Read the model definition and answer for the solid it produces. Units are mm, in the model's axes. Face numbers are marked on the shaded views. Round coordinates to 2 decimals unless told otherwise and drop trailing zeros. Order: outer loops, then holes, each group sorted by start corner. A loop starts at its lowest first (then second) coordinate and runs counter-clockwise, first axis right, second up. Notation, with made-up numbers: (22, 88.25) - (58, 88.25) arc R17 cw to (58, 110.25) - close; hole circle Ø6 at (72.25, 54.25). An arc over 180 degrees is marked (long way). Answer as a JSON object with one key per item and string values. Group by question number.
Q1. A cutting plane is placed at B-B on x = -9.5. Determine the outline of the cut face in (y, z), and give its area (3 significant figures).
Q2. The mould has two halves that part along Y. Classify the marked faces 1, 2 and 3: pulls with the +Y half, pulls with the -Y half, needs draft (parallel to the pull), parting line crosses it, or undercut.
Q3. A cutting plane is placed at D-D on z = 2.45. Determine the outline of the cut face in (x, y), and give its area (3 significant figures).
Q4. A cutting plane is placed at C-C on y = 1. Count the separate pieces of the cut face and the enclosed holes in it, and give its area (3 significant figures).
Q5. Consider line 1 (X direction, y = 0.5, z = 2.4); line 2 (Y direction, x = -15, z = 1.6); line 3 (X direction, y = 0.5, z = 1.15). Determine where each line is inside the solid, lowest interval first.
Q6. Given pin 1 Ø4 at (x, y) = (-15, 0) entering from -Z; pin 2 Ø2 at (x, y) = (0, 0) entering from +Z, each flat-ended and moving along its own axis, determine where each tip first touches the part or whether it passes through.
Q7. A cutting plane is placed at A-A on z = 1.55. Determine the outline of the cut face in (x, y), and give its area (3 significant figures).
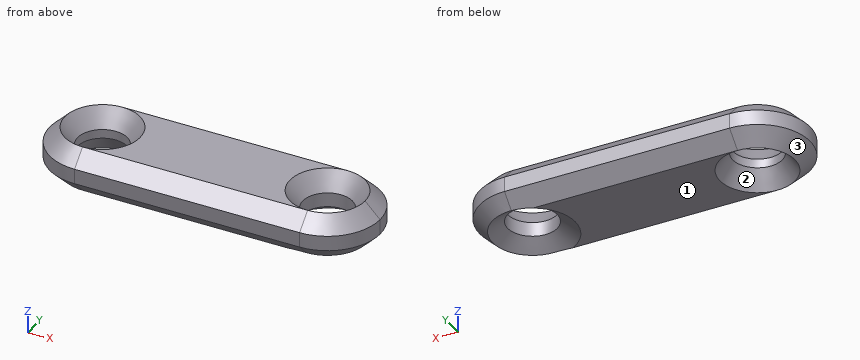
```python
from build123d import *

# Parameters (mm, degrees)
F0_R     = 1.65
F1_DEPTH = 3
F2_SIZE  = 1


# Not quite as in the source:
# - a fillet or chamfer that OpenCascade refuses, or shapes differently, is made with other operations: its cross-section is extruded or revolved along the edge and cut away or added


with BuildPart() as f1:
    # F0 (on Top) → F1 (new body)
    with BuildSketch(Plane.XY):
        with BuildLine():
            ThreePointArc((-15, -3.5), (-12.5251262658, -2.4748737342), (-11.5, 0))
            ThreePointArc((-11.5, 0), (-12.5251262658, 2.4748737342), (-15, 3.5))
            ThreePointArc((-15, 3.5), (-18.5, 0), (-15, -3.5))
        make_face()
        with Locations((-15, 0)):
            Circle(F0_R, mode=Mode.SUBTRACT)
        with BuildLine():
            ThreePointArc((-15, 3.5), (-12.5251262658, 2.4748737342), (-11.5, 0))
            ThreePointArc((-11.5, 0), (-12.5251262658, -2.4748737342), (-15, -3.5))
            Line((-15, -3.5), (0, -3.5))
            ThreePointArc((0, -3.5), (-3.5, 0), (0, 3.5))
            Line((0, 3.5), (-15, 3.5))
        make_face()
        with BuildLine():
            ThreePointArc((3.5, 0), (2.4748737342, 2.4748737342), (0, 3.5))
            ThreePointArc((0, 3.5), (-3.5, 0), (0, -3.5))
            ThreePointArc((0, -3.5), (2.4748737342, -2.4748737342), (3.5, 0))
        make_face()
        Circle(F0_R, mode=Mode.SUBTRACT)
    extrude(amount=F1_DEPTH)

    # F2
    f2_edges = [f1.edges().sort_by_distance(p)[0] for p in [
        (-7.5, -3.5, 3),
        (-18.5, 0, 3),
        (3.5, 0, 3),
        (-7.5, 3.5, 3),
        (-7.5, -3.5, 0),
        (-18.5, 0, 0),
        (3.5, 0, 0),
        (-7.5, 3.5, 0),
    ]]
    chamfer(f2_edges, length=F2_SIZE)

    # F3: chamfer of 1.2 x 0.85 on 4 edges, made by hand

    # F3_s1 → F3_t2 (revolve, cut)
    with BuildSketch(Plane.XZ):
        Polygon((-12.5, 3), (-13.35, 1.8), (-13.35, 3), align=None)
    revolve(axis=Axis((-15, 0, 3), (0, 0, 1)), mode=Mode.SUBTRACT)

    # F3_s3 → F3_t4 (revolve, cut)
    with BuildSketch(Plane.XZ):
        Polygon((2.5, 3), (1.65, 1.8), (1.65, 3), align=None)
    revolve(axis=Axis((0, 0, 3), (0, 0, 1)), mode=Mode.SUBTRACT)

    # F3_s5 → F3_t6 (revolve, cut)
    with BuildSketch(Plane.XZ):
        Polygon((2.85, 0), (1.65, 0.85), (1.65, 0), align=None)
    revolve(axis=Axis((0, 0, 0), (0, 0, 1)), mode=Mode.SUBTRACT)

    # F3_s7 → F3_t8 (revolve, cut)
    with BuildSketch(Plane.XZ):
        Polygon((-12.5, 0), (-13.35, 1.2), (-13.35, 0), align=None)
    revolve(axis=Axis((-15, 0, 0), (0, 0, 1)), mode=Mode.SUBTRACT)


solid = f1.part
```
Result set:
{
 "1": {"outline": "(-3.5, 1) - (-2.5, 0) - (2.5, 0) - (3.5, 1) - (3.5, 2) - (2.5, 3) - (-2.5, 3) - (-3.5, 2) - close", "area": "19.0 mm²"},
 "2": {"face 1": "needs draft", "face 2": "undercut", "face 3": "parting line crosses it"},
 "3": {"outline": "(-15, -3.05) - (0, -3.05) arc R3.05 ccw to (0, 3.05) - (-15, 3.05) arc R3.05 ccw to start; hole circle Ø4.22 at (-15, 0); hole circle Ø4.22 at (0, 0)", "area": "92.7 mm²"},
 "4": {"separate pieces": "3", "enclosed holes": "0", "area": "42.5 mm²"},
 "5": {"line 1": "x = -18.06 to -17.01, -12.99 to -2.01, 2.01 to 3.06", "line 2": "y = -3.5 to -1.65, 1.65 to 3.5", "line 3": "x = -18.46 to -16.61, -13.39 to -1.57, 1.57 to 3.46"},
 "6": {"pin 1": "stops at z = 0.71", "pin 2": "passes through"},
 "7": {"outline": "(-15, -3.5) - (0, -3.5) arc R3.5 ccw to (0, 3.5) - (-15, 3.5) arc R3.5 ccw to start; hole circle Ø3.3 at (-15, 0); hole circle Ø3.3 at (0, 0)", "area": "126 mm²"}
}
